Work out the finished part from the listing and answer in its coordinate system (mm). A direction names the side the tool comes from. Round coordinates to 2 decimals unless told otherwise and drop trailing zeros. Order: outer loops, then holes, each group sorted by start corner. A loop starts at its lowest first (then second) coordinate and runs counter-clockwise, first axis right, second up. Notation, with made-up numbers: (48.25, 73) - (96.25, 73) arc R32 cw to (96.25, 100) - close; hole circle Ø1 at (31, 60.5). An arc over 180 degrees is marked (long way). Put each result on its own line as item: value.
```python
from build123d import *

# Parameters (mm, degrees)
F0_W     = 98.9725068212
F0_H     = 67.7649602294
F1_DEPTH = 25.4
F2_DEPTH = 43.434
F3_DEPTH = 79.502
F4_R     = 15.6101521233
F5_DEPTH = 98.552
F7_DEPTH = 61.468
F9_DEPTH = 113.03


with BuildPart() as f1:
    # F0 (on Front) → F1 (new body)
    with BuildSketch(Plane.XZ):
        Polygon((57.0652261376, 41.9072769582), (-57.0652261376, 41.9072769582), (-57.0652261376, 25.8576832712), (41.9072806835, 25.8576832712), (41.9072806835, -41.9072769582), (57.0652261376, -41.9072769582), align=None)
        with Locations((-7.5789727271, -8.0247968435)):
            Rectangle(F0_W, F0_H)
    extrude(amount=F1_DEPTH)

    # F0 (on Front) → F2 (join)
    with BuildSketch(Plane.XZ):
        Polygon((57.0652261376, 41.9072769582), (-57.0652261376, 41.9072769582), (-57.0652261376, 25.8576832712), (41.9072806835, 25.8576832712), (41.9072806835, -41.9072769582), (57.0652261376, -41.9072769582), align=None)
    extrude(amount=F2_DEPTH)

    # F3 (add): a face of the model
    f3_faces = [f1.faces().sort_by_distance(p)[0] for p in [
        (-7.5789727271, -25.4, -8.0247968435),
    ]]
    extrude(f3_faces, amount=F3_DEPTH)

    # F4 (on face) → F5 (cut)
    with BuildSketch(Plane.YZ.offset(41.9072806835)):
        with Locations((-74.168, -8.0247968435)):
            Circle(F4_R)
    extrude(amount=-F5_DEPTH, mode=Mode.SUBTRACT)

    # F6 (on face) → F7 (cut)
    with BuildSketch(Plane.XZ.offset(104.902)):
        Polygon((-7.5789727271, 25.8576832712), (41.9072806835, -41.9072769582), (41.9072806835, 25.8576832712), align=None)
    extrude(amount=-F7_DEPTH, mode=Mode.SUBTRACT)

    # F8 (on Front) → F9 (cut, symmetric)
    with BuildSketch(Plane.XZ):
        Polygon((40.1673130691, 75.5145400763), (-28.9204549044, 49.1647869349), (43.7020324171, -55.2702136338), (114.3328375611, -6.154642004), align=None)
    extrude(amount=F9_DEPTH, both=True, mode=Mode.SUBTRACT)


solid = f1.part
```
1) Straight lines are drawn through the part: L1, parallel to Z at x = -40, y = -51; L2, parallel to Z at x = -11, y = -65.5; L3, parallel to X at y = -71, z = -20. For each, find the intervals that lie inside material, in ascending order. Write a range as from..to.
Findings below:
L1: z = -41.91..25.86
L2: z = -41.91..-21.01, 4.96..23.39
L3: x = -57.07..-56.64
2) A cutting plane is placed at D-D on x = 9.5. Write down the section's boundary in (y, z), then the cut area to 3 significant figures.
Findings below:
outline: (-104.9, -41.91) - (0, -41.91) - (0, -6.09) - (-58.68, -6.09) arc R15.61 cw (long way) to (-89.66, -6.09) - (-104.9, -6.09) - close
area: 3,310 mm2
3) A cutting plane is placed at A-A on z = -17.5. Write down the section's boundary in (x, y), then the cut area to 3 significant figures.
Findings below:
outline: (-57.07, -104.9) - (17.44, -104.9) - (17.44, -86.57) - (-56.64, -86.57) - (-56.64, -61.76) - (17.44, -61.76) - (17.44, 0) - (-57.07, 0) - close
area: 5,980 mm2
4) Given pin 1 Ø12 at (y, z) = (-58.5, 2) entering from +X; pin 2 Ø4 at (x, y) = (9.5, -21) entering from +Z; pin 3 Ø6 at (x, y) = (-14.5, -30.5) entering from +Z, each flat-ended and moving along its own axis, determine where each tip first touches the part or whether it passes through.
Findings below:
pin 1: stops at x = 8.05
pin 2: stops at z = -3.21
pin 3: stops at z = 32.74
5) For faces 1 (the cylindrical face through (-25.628, -77.552, -23.264)), 2 (the flat face through (-40, -21, 41.907)), determine the directions among +Z, -Z, +X, -X, +Y, -Y from which every point of the face is accessible in a straight line to the end or side of a thin tool.
Findings below:
face 1: +X
face 2: +Z, +X, -X, +Y, -Y
6) For a pull along Y with two mould halves and no side action, classify faces 3 (the flat face through (-22, 0, -9)), 4 (the flat face through (-56.645, -74, -8)), 5 (the flat face through (-40, -43.434, 34)), 6 (the flat face through (-35, -74, 25.858)) as pulls with the +Y half, pulls with the -Y half, needs draft (parallel to the pull), parting line crosses it, or undercut.
Findings below:
face 3: pulls with the +Y half
face 4: undercut
face 5: pulls with the -Y half
face 6: needs draft
7) A cutting plane is placed at B-B on x = -40.5. Write down the section's boundary in (y, z).
Findings below:
outline: (-104.9, -41.91) - (0, -41.91) - (0, 41.91) - (-43.43, 41.91) - (-43.43, 25.86) - (-104.9, 25.86) - close; hole circle Ø31.22 at (-74.17, -8.02)
8) A cutting plane is placed at C-C on y = -85. Write down the section's boundary in (x, z).
Findings below:
outline: (-57.07, -41.91) - (34.41, -41.91) - (18.66, -19.27) - (-56.64, -19.27) - (-56.64, 3.22) - (3.03, 3.22) - (-12.71, 25.86) - (-57.07, 25.86) - close
